from build123d import *

# Parameters (mm, degrees)
SKETCH1_W           = 304.8
SKETCH1_H           = 431.8
BOSS_EXTRUDE1_DEPTH = 431.8
SKETCH2_W           = 299.72
SKETCH2_H           = 426.72
CUT_EXTRUDE1_DEPTH  = 429.26
FILLET1_R           = 5.08
SKETCH3_W           = 33.02
SKETCH3_H           = 86.106
CUT_EXTRUDE2_DEPTH  = 3.54
SKETCH10_R          = 14.478
CUT_EXTRUDE7_DEPTH  = 7.62


with BuildPart() as part:
    # Sketch1 → Boss-Extrude1 (new body)
    with BuildSketch(Plane.XY):
        with Locations((152.4, 215.9)):
            Rectangle(SKETCH1_W, SKETCH1_H)
    extrude(amount=BOSS_EXTRUDE1_DEPTH)

    # Sketch2 → Cut-Extrude1 (cut)
    with BuildSketch(Plane(origin=(0, 431.8, 0), x_dir=(1, 0, 0), z_dir=(0, 1, 0))):
        with Locations((152.4, -215.9)):
            Rectangle(SKETCH2_W, SKETCH2_H)
    extrude(amount=-CUT_EXTRUDE1_DEPTH, mode=Mode.SUBTRACT)

    # Fillet1
    fillet1_edges = [part.edges().sort_by_distance(p)[0] for p in [
        (304.8, 215.9, 431.8),
        (0, 215.9, 431.8),
        (304.8, 215.9, 0),
        (152.4, 0, 0),
        (0, 215.9, 0),
        (304.8, 0, 215.9),
        (0, 0, 215.9),
        (152.4, 0, 431.8),
    ]]
    fillet(fillet1_edges, radius=FILLET1_R)

    # Sketch3 → Cut-Extrude2 (cut, through all)
    with BuildSketch(Plane(origin=(0, 2.54, 0), x_dir=(1, 0, 0), z_dir=(0, 1, 0))):
        with Locations((152.4, -370.967)):
            Rectangle(SKETCH3_W, SKETCH3_H)
    extrude(amount=-CUT_EXTRUDE2_DEPTH, mode=Mode.SUBTRACT)

    # Sketch10 → Cut-Extrude7 (cut)
    with BuildSketch(Plane.XY.offset(431.8)):
        with Locations((152.4, 21.59)):
            Circle(SKETCH10_R)
    extrude(amount=-CUT_EXTRUDE7_DEPTH, mode=Mode.SUBTRACT)


solid = part.part
Work out the finished part from the listing and answer in its coordinate system (mm). A direction names the side the tool comes from. Round coordinates to 2 decimals unless told otherwise and drop trailing zeros. Loops run counter-clockwise (first coordinate to the right, second up) from the corner with the lowest first, then second, coordinate; pieces in that order, holes last. Notation, with made-up numbers: M 15,24 L 42,24 A12 cw 42,46 Z; hole C 59.5,4.5 d8. An arc over 180 degrees is marked long. One line per question, with ' | ' between items. Start each with the question number.
(1) Flat-ended cylindrical pins translate along their axes: pin 1 Ø2 at (y, z) = (1, 362.5) entering from -X; pin 2 Ø2 at (y, z) = (1.5, 370.5) entering from +X; pin 3 Ø2 at (x, y) = (160.5, 1) entering from +Z. Find the tip coordinate at first contact, or state that the pin passes through.
(2) A cutting plane is placed at A-A on x = 152.4. Write down the section's boundary in (y, z).
(3) Find the intervals of material crossed by line 1 (Z direction, x = 38, y = 61); line 2 (X direction, y = 358.5, z = 336); line 3 (Y direction, x = 99, z = 23.5), in increasing order.
(4) A cutting plane is placed at B-B on z = 361.5. Write down the section's boundary in (x, y), plus the area to 3 significant figures.
(5) A cutting plane is placed at D-D on y = 21.59. Write down the section's boundary in (x, z), plus the area to 3 significant figures.
(6) A cutting plane is placed at C-C on y = 76.5. Write down the section's boundary in (x, z), plus the area to 3 significant figures.
(7) For a pull along X with two mould halves and no side action, classify faces 1 (the face through (0, 215, 213)), 2 (the face through (137.936, 22.227, 430.548)), 3 (the face through (150, 220, 2.54)), 4 (the face through (150, 221, 431.8)) as released by +X, released by -X, zero draft, split by the parting line, or undercut.
(8) A tool of negligible diameter and unlimited length cuts with its end or side. For faces 5 (the face through (302.26, 220, 219)), 6 (the face through (304.8, 215, 213)), from which of +Z, -Z, +X, -X, +Y, -Y can it reach the whole face along a straight path? Write none if from no direction.
Geometry check:
1) pin 1: stops at x = 1.04 | pin 2: stops at x = 304.1 | pin 3: stops at z = 430.76
2) outline: M 0,5.08 A5.08 ccw 5.08,0 L 431.8,0 L 431.8,2.54 L 2.54,2.54 L 2.54,327.91 L 0,327.91 Z; M 0,414.02 L 2.54,414.02 L 2.54,429.26 L 7.11,429.26 L 7.11,431.8 L 5.08,431.8 A5.08 ccw 0,426.72 Z; M 36.07,429.26 L 431.8,429.26 L 431.8,431.8 L 36.07,431.8 Z
3) line 1: z = 0 to 2.54, 429.26 to 431.8 | line 2: x = 0 to 2.54, 302.26 to 304.8 | line 3: y = 0 to 2.54
4) outline: M 0,5.08 A5.08 ccw 5.08,0 L 135.89,0 L 135.89,2.54 L 2.54,2.54 L 2.54,431.8 L 0,431.8 Z; M 168.91,0 L 299.72,0 A5.08 ccw 304.8,5.08 L 304.8,431.8 L 302.26,431.8 L 302.26,2.54 L 168.91,2.54 Z | area: 2,860 mm²
5) outline: M 0,5.08 A5.08 ccw 5.08,0 L 299.72,0 A5.08 ccw 304.8,5.08 L 304.8,426.72 A5.08 ccw 299.72,431.8 L 166.88,431.8 L 166.88,429.26 L 302.26,429.26 L 302.26,2.54 L 2.54,2.54 L 2.54,429.26 L 137.92,429.26 L 137.92,431.8 L 5.08,431.8 A5.08 ccw 0,426.72 Z | area: 3,620 mm²
6) outline: M 0,5.08 A5.08 ccw 5.08,0 L 299.72,0 A5.08 ccw 304.8,5.08 L 304.8,426.72 A5.08 ccw 299.72,431.8 L 5.08,431.8 A5.08 ccw 0,426.72 Z; hole M 2.54,2.54 L 302.26,2.54 L 302.26,429.26 L 2.54,429.26 Z | area: 3,690 mm²
7) face 1: released by -X | face 2: undercut | face 3: undercut | face 4: zero draft
8) face 5: +Y | face 6: +Z, -Z, +X, +Y, -Y
